Autodesk Inventor part; units mm, degrees
ref_plane "YZ Plane" through (0, 0, 0) normal (1, 0, 0) x (0, 1, 0)
ref_plane "XZ Plane" through (0, 0, 0) normal (0, 1, 0) x (-1, 0, 0)
ref_plane "XY Plane" through (0, 0, 0) normal (0, 0, 1) x (1, 0, 0)
sketch "Sketch1" plane through (0, 0, 0) normal (0, 1, 0) x (-1, 0, 0)
  line L0 (-10.5, 9.1) -> (10.5, 9.1)
  line L1 (10.5, 9.1) -> (10.5, -9.1)
  line L2 (10.5, -9.1) -> (-10.5, -9.1)
  line L3 (-10.5, -9.1) -> (-10.5, 9.1)
  line L4 (-10.5, 9.1) -> (10.5, -9.1) construction
  line L5 (10.5, 9.1) -> (-10.5, -9.1) construction
  line L6 (10.5, 9.1) -> (-10.5, 9.1)
  line L7 (-10.5, 9.1) -> (-10.5, 10.1)
  line L8 (-10.5, 10.1) -> (10.5, 10.1)
  line L9 (10.5, 10.1) -> (10.5, 9.1)
  line L10 (20.5, -26) -> (-10.5, -26)
  line L11 (-10.5, -26) -> (-10.5, -9.1)
  line L12 (-10.5, -9.1) -> (20.5, -9.1)
  line L13 (20.5, -9.1) -> (20.5, -26)
  circle A0 centre (10.5, -16) radius 3.5
  line L14 (-10.5, -9.1) -> (4.5, -26)
  circle A1 centre (6, -7.6) radius 1.15
  circle A2 centre (-7.5, -7.6) radius 1.15
  circle A3 centre (-7.5, 7.6) radius 1.15
  circle A4 centre (6, 7.6) radius 1.15
  circle A5 centre (-2.5, -14.1) radius 1.15
  circle A6 centre (-7.5, 0) radius 1.15
  point P0 (0, 0)
  point P1 (0, 0)
  point P2 (0, 0)
  point P3 (0, 0)
  dimension "d0" = 9.1
  dimension "d1" = 21
  dimension "d2" = 1
  dimension "d3" = 7
  dimension "d4" = 16
  dimension "d5" = 10
  dimension "d6" = 10
  dimension "d8" = 6
  dimension "d9" = 2.3
  dimension "d10" = 1.5
  dimension "d11" = 2.3
  dimension "d12" = 3
  dimension "d13" = 4.5
  dimension "d14" = 1.5
  dimension "d15" = 2.3
  dimension "d16" = 1.5
  dimension "d17" = 3
  dimension "d18" = 2.3
  dimension "d19" = 4.5
  dimension "d20" = 1.5
  dimension "d25" = 2.3
  dimension "d26" = 14.1
  dimension "d27" = 8
  dimension "d28" = 2.3
  dimension "d29" = 3
extrude "Extrusion1" add sketch "Sketch1" along normal blind 3 contours L7 L8 L9 L0 | L0 L1 L2 L3 | L2 L12 L13 L10 L14
fillet "Fillet1" radius 2 4 edges at (-10.5, 1.5, -9.1) (10.5, 1.5, -9.1) (10.5, 1.5, 10.1) (-10.5, 1.5, 10.1)
fillet "Fillet2" radius 6 3 edges at (-20.5, 1.5, -9.1) (-20.5, 1.5, -26) (-4.5, 1.5, -26)
sketch "Sketch2" plane through (0, 3, 0) normal (0, 1, 0) x (1, 0, 0)
  arc A0 (-2.7097, 23.9829) -> (-7.197, 26) centre (-7.197, 20) ccw
  line L0 (-7.197, 26) -> (-14.5, 26)
  arc A1 (-14.5, 26) -> (-20.5, 20) centre (-14.5, 20) ccw
  line L1 (-20.5, 20) -> (-20.5, 15.1)
  arc A2 (-20.5, 15.1) -> (-14.5, 9.1) centre (-14.5, 15.1) ccw
  line L2 (-14.5, 9.1) -> (-12.5, 9.1)
  arc A3 (-10.5, 7.1) -> (-12.5, 9.1) centre (-12.5, 7.1) ccw
  line L3 (-10.5, 7.1) -> (-10.5, -8.1)
  arc A4 (-10.5, -8.1) -> (-8.5, -10.1) centre (-8.5, -8.1) ccw
  line L4 (-8.5, -10.1) -> (8.5, -10.1)
  arc A5 (8.5, -10.1) -> (10.5, -8.1) centre (8.5, -8.1) ccw
  line L5 (10.5, -8.1) -> (10.5, 8.3404)
  arc A6 (10.5, 8.3404) -> (9.9958, 9.6681) centre (8.5, 8.3404) ccw
  line L6 (9.9958, 9.6681) -> (-2.7097, 23.9829)
  circle A7 centre (2.5, 14.1) radius 1.15
  circle A8 centre (-10.5, 16) radius 3.5
  circle A9 centre (-6, 7.6) radius 1.15
  circle A10 centre (7.5, 7.6) radius 1.15
  circle A11 centre (7.5, -7.6) radius 1.15
  circle A12 centre (-6, -7.6) radius 1.15
  circle A13 centre (7.5, 0) radius 1.15
  point P0 (0, 0)
properties part number "New_hinge_plate"
CAD build for the part. Positions are in the model's coordinates, mm. Coordinates: 2 decimals unless noted, no trailing zeros. Order: outer loops, then holes, each group sorted by start corner. A loop starts at its lowest first (then second) coordinate and runs counter-clockwise, first axis right, second up. Notation, with made-up numbers: (56, 23.25) - (111, 23.25) arc R18 cw to (111, 54.25) - close; hole circle Ø2 at (61.5, 40.5). An arc over 180 degrees is marked (long way). Answer in a Markdown table with one row per item.
1. Slice it at A-A, the plane z = 7.6. List the corners of the cut face in (x, y), then the cut area to 3 significant figures.
Answer:
| item | result |
|---|---|
| outline | (-10.5, 0) - (-7.15, 0) - (-7.15, 3) - (-10.5, 3) - close; (-4.85, 0) - (6.35, 0) - (6.35, 3) - (-4.85, 3) - close; (8.65, 0) - (10.5, 0) - (10.5, 3) - (8.65, 3) - close |
| area | 49.2 mm² |
2. Slice it at B-B, the plane y = 1.1. List the corners of the cut face in (x, z).
Answer:
| item | result |
|---|---|
| outline | (-20.5, -20) arc R6 ccw to (-14.5, -26) - (-7.2, -26) arc R6 ccw to (-2.71, -23.98) - (10, -9.67) arc R2 ccw to (10.5, -8.34) - (10.5, 8.1) arc R2 ccw to (8.5, 10.1) - (-8.5, 10.1) arc R2 ccw to (-10.5, 8.1) - (-10.5, -7.1) arc R2 cw to (-12.5, -9.1) - (-14.5, -9.1) arc R6 ccw to (-20.5, -15.1) - close; hole circle Ø7 at (-10.5, -16); hole circle Ø2.3 at (-6, -7.6); hole circle Ø2.3 at (-6, 7.6); hole circle Ø2.3 at (2.5, -14.1); hole circle Ø2.3 at (7.5, -7.6); hole circle Ø2.3 at (7.5, 0); hole circle Ø2.3 at (7.5, 7.6) |
3. Slice it at D-D, the plane x = 8. List the corners of the cut face in (y, z).
Answer:
| item | result |
|---|---|
| outline | (0, -11.92) - (3, -11.92) - (3, -8.64) - (0, -8.64) - close; (0, -6.56) - (3, -6.56) - (3, -1.04) - (0, -1.04) - close; (0, 1.04) - (3, 1.04) - (3, 6.56) - (0, 6.56) - close; (0, 8.64) - (3, 8.64) - (3, 10.1) - (0, 10.1) - close |
4. Drill centre lines: L1, parallel to Z at x = 7.5, y = 1.4; L2, parallel to X at y = 0.55, z = -7; L3, parallel to Z at x = -6, y = 1.05. Where is each one in solid material? Low to high. Write a range as from..to.
Answer:
| item | result |
|---|---|
| L1 | -12.48..-8.75, -6.45..-1.15, 1.15..6.45, 8.75..10.1 |
| L2 | -10.5..-6.98, -5.02..6.52, 8.48..10.5 |
| L3 | -25.88..-8.75, -6.45..6.45, 8.75..10.1 |
5. Slice it at C-C, the plane z = 0. List the corners of the cut face in (x, y), then the cut area to 3 significant figures.
Answer:
| item | result |
|---|---|
| outline | (-10.5, 0) - (6.35, 0) - (6.35, 3) - (-10.5, 3) - close; (8.65, 0) - (10.5, 0) - (10.5, 3) - (8.65, 3) - close |
| area | 56.1 mm² |
6. Flat gauge pins, fed straight in: P1, Ø1.4, axis at x = 2.5, z = -14.1, coming from the -Y side; P2, Ø1, axis at x = -13.5, y = 1, coming from the +Z side. Where does each tip first touch, or does it go through?
Answer:
| item | result |
|---|---|
| P1 | through |
| P2 | z = -9.1 |
7. Pull direction Z, two halves, no side cores. Call faces 1 (the face through (-10.5, 1, 1)), 2 (the face through (-5.09, 1.48, 8.3)), 3 (the face through (2.749, 1.479, -12.977)), 4 (the face through (-4.705, 1.521, -25.458)): +Z half, -Z half, draft (parallel to the pull), parting line (faces both ways), or undercut.
Answer:
| item | result |
|---|---|
| face 1 | draft |
| face 2 | undercut |
| face 3 | undercut |
| face 4 | -Z half |
